Can you work these out from the model? Positions are in its coordinate system, mm. Face numbers are marked on the shaded views. A direction names the side the tool comes from. Give positions to 0.01 mm unless a question says otherwise; leave off trailing zeros. Loops run counter-clockwise (first coordinate to the right, second up) from the corner with the lowest first, then second, coordinate; pieces in that order, holes last. Notation, with made-up numbers: M 36,-31 L 62,-31 A21 cw 62,6 Z; hole C 78.5,-38.75 d11. An arc over 180 degrees is marked long. Put each result on its own line as item: value. Start each with the question number.
1) For the marked faces 1, 2, 3 and 4, which set-ups out of +Z, -Z, +X, -X, +Y, -Y let a thin tool reach every point of the face, with its end or its side?
2) Imagine slicing it at A-A (y = -61.15). Write out the boundary of the cut face in (x, z).
3) Please list where these lines run through material, in increasing order: line 1 along Y through (x, z) = (-8.2, -65.15); line 2 along Z through (x, y) = (-27.15, -50); line 3 along Z through (x, y) = (-15.75, -71.5). Write a range as from..to.
4) Imagine slicing it at D-D (y = -46). Write out the boundary of the cut face in (x, z), then the cut area to 3 significant figures.
5) For P1, Ø1.2, axis at x = -27, z = -33, coming from the -Y side; P2, Ø1, axis at x = -18, y = -52, coming from the +Z side; P3, Ø5, axis at x = -20.5, y = -93, coming from the -Z side, each with a flat end and sliding along its axis, tell me the tip position at first contact or that it passes through.
6) Imagine slicing it at B-B (z = -30). Write out the boundary of the cut face in (x, y), then the cut area to 3 significant figures.
7) Imagine slicing it at C-C (z = -65.15). Write out the boundary of the cut face in (x, y).
from build123d import *

# Parameters (mm, degrees)
SKICA2_W                 = 20
SKICA2_H                 = 42.3
P_IDAT_VYSUNUT_M1_DEPTH  = 4
SKICA3_W                 = 24
SKICA3_H                 = 42.3
P_IDAT_VYSUNUT_M2_DEPTH  = 4
SKICA4_W                 = 6
SKICA4_H                 = 42.3
P_IDAT_VYSUNUT_M3_DEPTH  = 42.3
SKICA5_R                 = 11.05
ODEBRAT_VYSUNUT_M1_DEPTH = 7
SKICA7_R                 = 2.6
ODEBRAT_VYSUNUT_M3_DEPTH = 4
ZKOSEN_1_SIZE            = 1
SKICA8_W                 = 20
SKICA8_H                 = 4
P_IDAT_VYSUNUT_M4_DEPTH  = 20.091596743
SKICA9_R                 = 2.6
ODEBRAT_VYSUNUT_M4_DEPTH = 4
ODEBRAT_VYSUNUT_M5_DEPTH = 80
SKICA11_W                = 84.692176523
SKICA11_H                = 80.474242756
ODEBRAT_VYSUNUT_M6_DEPTH = 24


with BuildPart() as part:
    # Skica2 → Přidat vysunutím1 (new body)
    with BuildSketch(Plane.XY):
        with Locations((-14.524287798, -61.15)):
            Rectangle(SKICA2_W, SKICA2_H)
    extrude(amount=P_IDAT_VYSUNUT_M1_DEPTH)

    # Skica3 → Přidat vysunutím2 (add)
    with BuildSketch(Plane.ZY.offset(24.524287798)):
        with Locations((-8, -61.15)):
            Rectangle(SKICA3_W, SKICA3_H)
    extrude(amount=P_IDAT_VYSUNUT_M2_DEPTH)

    # Skica4 → Přidat vysunutím3 (add)
    with BuildSketch(Plane.XY.offset(4)):
        with Locations((-7.524287798, -61.15)):
            Rectangle(SKICA4_W, SKICA4_H)
    extrude(amount=P_IDAT_VYSUNUT_M3_DEPTH)

    # Skica5 → Odebrat vysunutím1 (cut)
    with BuildSketch(Plane(origin=(-4.524287798, 0, 0), x_dir=(0, 0, -1), z_dir=(1, 0, 0))):
        with Locations((-25.15, -61.15)):
            Circle(SKICA5_R)
    extrude(amount=-ODEBRAT_VYSUNUT_M1_DEPTH, mode=Mode.SUBTRACT)

    # Skica7 → Odebrat vysunutím3 (cut)
    with BuildSketch(Plane.ZY.offset(28.524287798)):
        with Locations(Location((-10, -50, 0), (0, 0, 270))):
            Circle(SKICA7_R)
        with Locations(Location((-10, -70, 0), (0, 0, 270))):
            Circle(SKICA7_R)
    extrude(amount=-ODEBRAT_VYSUNUT_M3_DEPTH, mode=Mode.SUBTRACT)

    # Zkosení1
    zkosen_1_edges = [part.edges().sort_by_distance(p)[0] for p in [
        (-10.524287798, -61.15, 36.2),
    ]]
    chamfer(zkosen_1_edges, length=ZKOSEN_1_SIZE)

    # Skica8 → Přidat vysunutím4 (add)
    with BuildSketch(Plane.XZ.offset(82.3)):
        with Locations((-14.524287798, 2)):
            Rectangle(SKICA8_W, SKICA8_H)
    extrude(amount=P_IDAT_VYSUNUT_M4_DEPTH)

    # Skica9 → Odebrat vysunutím4 (cut)
    with BuildSketch(Plane.XY.offset(4)):
        with Locations((-14.524287798, -92.391596743)):
            Circle(SKICA9_R)
    extrude(amount=-ODEBRAT_VYSUNUT_M4_DEPTH, mode=Mode.SUBTRACT)

    # Skica10 → Odebrat vysunutím5 (cut)
    with BuildSketch(Plane.ZY.offset(10.524287798)):
        Polygon((46.3, -44), (42.3, -40), (46.565878614, -39.259270079), align=None)
        Polygon((42.3, -82.3), (46.3, -78.3), (47.745576453, -80.3), (46.3, -85.415433185), align=None)
    extrude(amount=-ODEBRAT_VYSUNUT_M5_DEPTH, mode=Mode.SUBTRACT)


with BuildPart() as body_2:
    # Zrcadlit1: mirrored copy
    add(part.part.mirror(Plane(origin=(-28.524287798, -40, -20), x_dir=(1, 0, 0), z_dir=(0, 0, 1))))


with BuildPart() as part_1:
    add(part.part)

    # Skica11 → Odebrat vysunutím6 (cut)
    with BuildSketch(Plane.ZY.offset(28.524287798)):
        with Locations((22.346088262, -80.237121378)):
            Rectangle(SKICA11_W, SKICA11_H)
    extrude(amount=-ODEBRAT_VYSUNUT_M6_DEPTH, mode=Mode.SUBTRACT)


solid = body_2.part
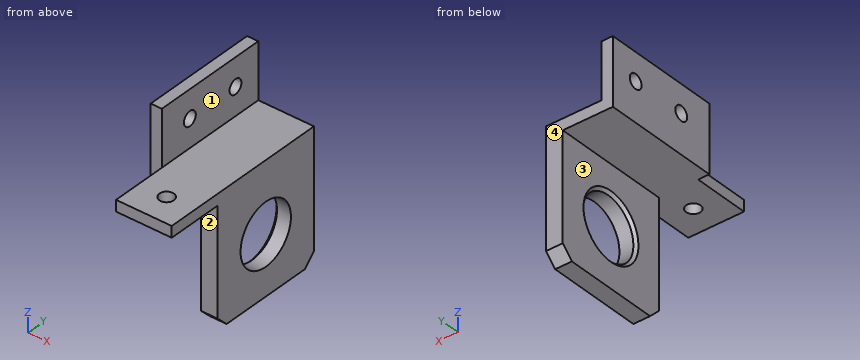
Recorded:
1. face 1: +Z, +X, +Y, -Y
1. face 2: -Z, +X, -X, -Y
1. face 3: -Z, -X, +Y, -Y
1. face 4: +Z, -Z, +X, -X, +Y
2. outline: M -28.52,-44 L -10.52,-44 L -10.52,-53.1 L -9.52,-54.1 L -4.52,-54.1 L -4.52,-40 L -24.52,-40 L -24.52,-20 L -28.52,-20 Z; M -10.52,-86.3 L -4.52,-86.3 L -4.52,-76.2 L -9.52,-76.2 L -10.52,-77.2 Z
3. line 1: -82.3..-72.2, -50.1..-40
3. line 2: -44..-32.6, -27.4..-20
3. line 3: -44..-40
4. outline: M -28.52,-44 L -10.52,-44 L -10.52,-86.3 L -4.52,-86.3 L -4.52,-40 L -24.52,-40 L -24.52,-20 L -28.52,-20 Z
4. area: 430 mm²
5. P1: y = -82.3
5. P2: z = -40
5. P3: z = -44
6. outline: M -28.52,-82.3 L -24.52,-82.3 L -24.52,-72.6 L -28.52,-72.6 Z; M -28.52,-67.4 L -24.52,-67.4 L -24.52,-52.6 L -28.52,-52.6 Z; M -28.52,-47.4 L -24.52,-47.4 L -24.52,-40 L -28.52,-40 Z
6. area: 128 mm²
7. outline: M -10.52,-82.3 L -4.52,-82.3 L -4.52,-72.2 L -9.52,-72.2 L -10.52,-73.2 Z; M -10.52,-49.1 L -9.52,-50.1 L -4.52,-50.1 L -4.52,-40 L -10.52,-40 Z
